```python
from build123d import *

# Parameters (mm, degrees)
SKETCH1_R           = 10
BOSS_EXTRUDE1_DEPTH = 2
SKETCH2_R           = 1
SKETCH2_W           = 2
SKETCH2_H           = 5
CUT_EXTRUDE1_DEPTH  = 2
SKETCH3_R           = 3.2
CUT_EXTRUDE2_DEPTH  = 0.2


with BuildPart() as part:
    # Sketch1 → Boss-Extrude1 (new body)
    with BuildSketch(Plane(origin=(0, 0, 0), x_dir=(1, 0, 0), z_dir=(0, 1, 0))):
        with Locations(Location((0, 0, 0), (0, 0, 270))):
            Circle(SKETCH1_R)
    extrude(amount=BOSS_EXTRUDE1_DEPTH)

    # Sketch2 → Cut-Extrude1 (cut)
    with BuildSketch(Plane(origin=(0, 2, 0), x_dir=(1, 0, 0), z_dir=(0, 1, 0))):
        with Locations(Location((0, 0, 0), (0, 0, 270))):
            Circle(SKETCH2_R)
        with Locations(Location((5, 0, 0), (0, 0, 270))):
            Circle(SKETCH2_R)
        with Locations(Location((-5, 0, 0), (0, 0, 90))):
            Circle(SKETCH2_R)
        with Locations((0, 4)):
            Rectangle(SKETCH2_W, SKETCH2_H)
    extrude(amount=-CUT_EXTRUDE1_DEPTH, mode=Mode.SUBTRACT)

    # Sketch3 → Cut-Extrude2 (cut)
    with BuildSketch(Plane.XZ):
        Circle(SKETCH3_R)
    extrude(amount=-CUT_EXTRUDE2_DEPTH, mode=Mode.SUBTRACT)


solid = part.part
```
For this review, take the finished solid that the model builds, in its own axes (mm). A direction names the side the tool comes from. Round coordinates to 2 decimals unless told otherwise and drop trailing zeros. Write each loop counter-clockwise with the first axis right and the second up, starting at its lowest first coordinate (ties: lowest second). Pieces come first, ordered by that corner, then holes. Notation, with made-up numbers: M -2.5,16 L 54.5,16 A17 cw 54.5,27 Z; hole C -28.5,-32 d2. An arc over 180 degrees is marked long. One line per item, written item: value. Start each with the question number.
(1) We need section B-B (z = 0). Give the boundary of the cut face in (x, y).
(2) Insertion check: pin 1 (1 mm diameter, centred on y = 1, z = -5, fed in from -X); pin 2 (1.8 mm diameter, centred on x = 0, z = 0, fed in from +Y). Each pin has a flat end and moves straight along its axis. Give the tip position at first contact, or say it passes through.
(3) Machinability: for faces 5 (the flat face through (0, 1, -6.5)), 6 (the flat face through (2.4, 0, -2.4)), 7 (the flat face through (1, 0.2, 1)), which of the approach directions +Z, -Z, +X, -X, +Y, -Y give a long, thin tool a straight path to every point of the face, cutting with its end or side? Answer none if there is none.
(4) Wall thickness on line 1 (X direction, y = 0.5, z = 0); line 2 (X direction, y = 0.1, z = 0); line 3 (X direction, y = 0.1, z = -4.25): over which ranges is each line inside the solid? List them lowest first.
(5) We need section D-D (z = -5.25). Give the boundary of the cut face in (x, y), and give its area (3 significant figures).
(6) We need section A-A (x = 0). Give the boundary of the cut face in (y, z).
(7) The part is to be moulded in two halves that separate along Z. For faces 1 (the flat face through (1, 1, -4)), 2 (the flat face through (0, 2, 2)), 3 (the cylindrical face through (-9.76, 0.99, -2.17)), 4 (the flat face through (0, 1, -1.5)), say which applies: released by +Z, released by -Z, zero draft, split by the parting line, or undercut.
(8) We need section C-C (y = 0.95). Give the boundary of the cut face in (x, z).
Result:
1. outline: M -10,0 L -6,0 L -6,2 L -10,2 Z; M -4,0 L -3.2,0 L -3.2,0.2 L -1,0.2 L -1,2 L -4,2 Z; M 1,0.2 L 3.2,0.2 L 3.2,0 L 4,0 L 4,2 L 1,2 Z; M 6,0 L 10,0 L 10,2 L 6,2 Z
2. pin 1: x = -8.93
2. pin 2: through
3. face 5: +Y, -Y
3. face 6: +Z, -Z, +X, -X, -Y
3. face 7: -Y
4. line 1: -10 to -6, -4 to -1, 1 to 4, 6 to 10
4. line 2: -10 to -6, -4 to -3.2, 3.2 to 4, 6 to 10
4. line 3: -9.05 to -1, 1 to 9.05
5. outline: M -8.51,0 L -1,0 L -1,2 L -8.51,2 Z; M 1,0 L 8.51,0 L 8.51,2 L 1,2 Z
5. area: 30.0 mm²
6. outline: M 0,-10 L 2,-10 L 2,-6.5 L 0,-6.5 Z; M 0,3.2 L 0.2,3.2 L 0.2,1 L 2,1 L 2,10 L 0,10 Z; M 0.2,-1.5 L 2,-1.5 L 2,-1 L 0.2,-1 Z
7. face 1: undercut
7. face 2: zero draft
7. face 3: split by the parting line
7. face 4: undercut
8. outline: C 0,0 d20; hole C -5,0 d2; hole M -1,-6.5 L 1,-6.5 L 1,-1.5 L -1,-1.5 Z; hole C 0,0 d2; hole C 5,0 d2
